```python
from build123d import *

# Parameters (mm, degrees)
SKETCH1_R           = 2.4892
BOSS_EXTRUDE1_DEPTH = 3.175


with BuildPart() as part:
    # Sketch1 → Boss-Extrude1 (new, symmetric)
    with BuildSketch(Plane.XY):
        with BuildLine():
            Line((-6.35, 27.3812), (-44.45, 27.3812))
            Line((-44.45, 27.3812), (-44.45, -48.8188))
            Line((-44.45, -48.8188), (-10.31875, -48.8188))
            Line((-10.31875, -48.8188), (-10.31875, -15.734319794))
            ThreePointArc((-10.31875, -15.734319794), (-10.89585042, -11.492870345), (-12.585193267, -7.559797873))
            ThreePointArc((-12.585193267, -7.559797873), (-14.062748456, 4.216247062), (-6.35, 13.236885338))
            Line((-6.35, 13.236885338), (-6.35, 27.3812))
        make_face()
        with Locations((-31.75, 14.6812)):
            Circle(SKETCH1_R, mode=Mode.SUBTRACT)
        with Locations((-31.75, -36.1188)):
            Circle(SKETCH1_R, mode=Mode.SUBTRACT)
    extrude(amount=BOSS_EXTRUDE1_DEPTH, both=True)


solid = part.part
```
Geometry check sheet. Reference: the model listing, model coordinates, mm. A direction names the side the tool comes from. Coordinates: 2 decimals unless noted, no trailing zeros. Order: outer loops, then holes, each group sorted by start corner. A loop starts at its lowest first (then second) coordinate and runs counter-clockwise, first axis right, second up. Notation, with made-up numbers: M 6.5,53 L 59.5,53 A15 ccw 59.5,80 Z; hole C 85.25,37 d2. An arc over 180 degrees is marked long. Answer as a JSON object with one key per item and string values.
Q1. Cross-section at A-A on x = -31.75. Record the cut outline in (y, z) (3 decimals).
Results are:
{"outline": "M -48.819,-3.175 L -38.608,-3.175 L -38.608,3.175 L -48.819,3.175 Z; M -33.63,-3.175 L 12.192,-3.175 L 12.192,3.175 L -33.63,3.175 Z; M 17.17,-3.175 L 27.381,-3.175 L 27.381,3.175 L 17.17,3.175 Z"}
Q2. Tool access check on faces 5 (the flat face through (-25, 27.381, 0)), 6 (the flat face through (-10.319, -33, 0)). Record the directions out of +Z, -Z, +X, -X, +Y, -Y that give a thin tool (end or side, any length) a straight path to the whole face; none if there is none.
Results are:
{"face 5": "+Z, -Z, +X, -X, +Y", "face 6": "+Z, -Z, +X, -Y"}
Q3. Cross-section at C-C on y = -41.5. Record the cut outline in (x, z) (3 decimals).
Results are:
{"outline": "M -44.45,-3.175 L -10.319,-3.175 L -10.319,3.175 L -44.45,3.175 Z"}
Q4. Scan lines: line 1 (Y direction, x = -31.5, z = 2.75); line 2 (X direction, y = -40.5, z = -2.5); line 3 (Y direction, x = -33, z = -0.75). Record each from-to range of solid material in increasing order.
Results are:
{"line 1": "y = -48.82 to -38.6, -33.64 to 12.2, 17.16 to 27.38", "line 2": "x = -44.45 to -10.32", "line 3": "y = -48.82 to -38.27, -33.97 to 12.53, 16.83 to 27.38"}
Q5. Cross-section at B-B on z = -0.25. Record the cut outline in (x, y) (3 decimals), and give its area (3 significant figures).
Results are:
{"outline": "M -44.45,-48.819 L -10.319,-48.819 L -10.319,-15.734 A15.875 ccw -12.585,-7.56 A14.681 cw -6.35,13.237 L -6.35,27.381 L -44.45,27.381 Z; hole C -31.75,-36.119 d4.978; hole C -31.75,14.681 d4.978", "area": "2,560 mm²"}
Q6. Depth check by flat-ended pin: pin 1 Ø2 at (y, z) = (10, -1.5) entering from +X. Enter the tip coordinate at first touch or a pass-through.
Results are:
{"pin 1": "stops at x = -9.72"}
Q7. Release check for a two-part mould opening along X. For faces 1 (the cylindrical face through (-32.29, -38.55, -0.04)), 2 (the cylindrical face through (-33.73, 13.17, -0.04)), 3 (the flat face through (-26, -10, 3.175)), 4 (the cylindrical face through (-10.88, -11.55, 0.04)) record: released by +X, released by -X, zero draft, split by the parting line, or undercut.
Results are:
{"face 1": "undercut", "face 2": "undercut", "face 3": "zero draft", "face 4": "released by +X"}
